Check sheet for the modelled part. Datum: model origin and axes. Units: mm. A direction names the side the tool comes from. Give positions to 0.01 mm unless a question says otherwise; leave off trailing zeros. Order: outer loops, then holes, each group sorted by start corner. A loop starts at its lowest first (then second) coordinate and runs counter-clockwise, first axis right, second up.
Item 1: Sectioned sample at B-B on x = 38.5. Record the boundary of the cut face in (y, z).
Item 2: Sectioned sample at C-C on z = -4. Record the boundary of the cut face in (x, y).
Item 3: Access from +Z, -Z, +X, -X, +Y, -Y to the whole of each face (thin tool, end or side, straight path). Record for faces 1 (the cylindrical face through (18.78, -7.57, 0.27)), 2 (the cylindrical face through (-39.7, 5.6, 0.1)).
Item 4: Sectioned sample at D-D on x = 20. Record the boundary of the cut face in (y, z).
Item 5: Material ranges on line 1 along X through (y, z) = (-7, 4.5); line 2 along Y through (x, z) = (38.5, -3); line 3 along X through (y, z) = (-10, 1), recorded low to high.
Item 6: Sectioned sample at A-A on y = 6.5. Record the boundary of the cut face in (x, z), and give its area (3 significant figures).
Item 7: Release check for a two-part mould opening along Y. For faces 3 (the cylindrical face through (-39.7, -7.4, 0.1)), 4 (the cylindrical face through (37.3, 5.6, 0.1)), 5 (the flat face through (-1, -12.5, 0)), 6 (the flat face through (-1, 0, 5)) record: released by +Y, released by -Y, zero draft, split by the parting line, or undercut.
Item 8: Gauge pin test, flat ends, axial feed: P1, Ø2.5, axis at x = 38.5, y = -6.5, coming from the -Z side; P2, Ø1.5, axis at x = 20, z = 0, coming from the -Y side. Record the tip position at first contact, or that the pin passes through.
from build123d import *

# Parameters (mm, degrees)
EXTRUDE_383_DEPTH      = 5
EXTRUDE_383_DEPTH_BACK = 5
SKETCH_1_W             = 85
SKETCH_1_H             = 25
SKETCH_4_R             = 1.5
CUT_EXTRUDE_595_DEPTH  = 46.414755311
SKETCH_6_R             = 1.25
CUT_EXTRUDE_761_DEPTH  = 10
FILLET_2_R             = 5


with BuildPart() as part:
    # Sketch 1 → Extrude 383 (new, two sides: drawn at the far end of the back side and taken through both)
    with BuildSketch(Plane.XY.offset(-EXTRUDE_383_DEPTH_BACK)):
        Rectangle(SKETCH_1_W, SKETCH_1_H)
    extrude(amount=EXTRUDE_383_DEPTH + EXTRUDE_383_DEPTH_BACK)

    # Sketch 4 → Cut-Extrude 595 (cut, through all)
    with BuildSketch(Plane.XY.offset(5)):
        with Locations((-38.5, 6.5)):
            Circle(SKETCH_4_R)
        with Locations((38.5, 6.5)):
            Circle(SKETCH_4_R)
        with Locations((38.5, -6.5)):
            Circle(SKETCH_4_R)
        with Locations((-38.5, -6.5)):
            Circle(SKETCH_4_R)
    extrude(amount=-CUT_EXTRUDE_595_DEPTH, mode=Mode.SUBTRACT)

    # Sketch 6 → Cut-Extrude 761 (cut)
    with BuildSketch(Plane.XZ.offset(12.5)):
        with Locations(Location((-20, 0, 0), (0, 0, 270))):
            Circle(SKETCH_6_R)
        with Locations(Location((20, 0, 0), (0, 0, 270))):
            Circle(SKETCH_6_R)
    extrude(amount=-CUT_EXTRUDE_761_DEPTH, mode=Mode.SUBTRACT)

    # Fillet 2
    fillet_2_edges = [part.edges().sort_by_distance(p)[0] for p in [
        (-42.5, 12.5, 0),
        (42.5, 12.5, 0),
    ]]
    fillet(fillet_2_edges, radius=FILLET_2_R)


solid = part.part
Report:
1. outline: (-12.5, -5) - (-8, -5) - (-8, 5) - (-12.5, 5) - close; (-5, -5) - (5, -5) - (5, 5) - (-5, 5) - close; (8, -5) - (12.4, -5) - (12.4, 5) - (8, 5) - close
2. outline: (-42.5, -12.5) - (42.5, -12.5) - (42.5, 7.5) arc R5 ccw to (37.5, 12.5) - (-37.5, 12.5) arc R5 ccw to (-42.5, 7.5) - close; hole circle Ø3 at (-38.5, -6.5); hole circle Ø3 at (-38.5, 6.5); hole circle Ø3 at (38.5, -6.5); hole circle Ø3 at (38.5, 6.5)
3. face 1: -Y
3. face 2: +Z, -Z
4. outline: (-12.5, -5) - (12.5, -5) - (12.5, 5) - (-12.5, 5) - (-12.5, 1.25) - (-2.5, 1.25) - (-2.5, -1.25) - (-12.5, -1.25) - close
5. line 1: x = -42.5 to -39.91, -37.09 to 37.09, 39.91 to 42.5
5. line 2: y = -12.5 to -8, -5 to 5, 8 to 12.4
5. line 3: x = -42.5 to -20.75, -19.25 to 19.25, 20.75 to 42.5
6. outline: (-42.5, -5) - (-40, -5) - (-40, 5) - (-42.5, 5) - close; (-37, -5) - (37, -5) - (37, 5) - (-37, 5) - close; (40, -5) - (42.5, -5) - (42.5, 5) - (40, 5) - close
6. area: 790 mm2
7. face 3: undercut
7. face 4: undercut
7. face 5: released by -Y
7. face 6: zero draft
8. P1: passes through
8. P2: stops at y = -2.5
